from build123d import *

# Parameters (mm, degrees)
SKETCH1_W                = 10
SKETCH1_H                = 18
BOSS_EXTRUDE1_DEPTH      = 10
BOSS_EXTRUDE1_DEPTH_BACK = 10
SKETCH2_W                = 20
SKETCH2_H                = 2
BOSS_EXTRUDE2_DEPTH      = 20
SKETCH3_W                = 7
SKETCH3_H                = 4
SKETCH3_H_2              = 3
BOSS_EXTRUDE3_DEPTH      = 40
SKETCH7_R                = 1.5
CUT_EXTRUDE2_DEPTH       = 10


with BuildPart() as part:
    # Sketch1 → Boss-Extrude1 (new body, two sides)
    with BuildSketch(Plane.XY) as boss_extrude1_sk:
        with Locations((0, 6)):
            Rectangle(SKETCH1_W, SKETCH1_H)
    extrude(amount=BOSS_EXTRUDE1_DEPTH)
    extrude(boss_extrude1_sk.sketch, amount=-BOSS_EXTRUDE1_DEPTH_BACK)

    # Sketch2 → Boss-Extrude2 (add)
    with BuildSketch(Plane(origin=(0, 0, 0), x_dir=(0, 0, -1), z_dir=(1, 0, 0))):
        with Locations((0, -2)):
            Rectangle(SKETCH2_W, SKETCH2_H)
    extrude(amount=-BOSS_EXTRUDE2_DEPTH)

    # Sketch3 → Boss-Extrude3 (add)
    with BuildSketch(Plane(origin=(0, 0, 0), x_dir=(0, 0, -1), z_dir=(1, 0, 0))):
        with Locations((-6.5, 13)):
            Rectangle(SKETCH3_W, SKETCH3_H)
        with Locations((-6.5, -1.5)):
            Rectangle(SKETCH3_W, SKETCH3_H_2)
        with Locations((6.5, -1.5)):
            Rectangle(SKETCH3_W, SKETCH3_H_2)
        with Locations((6.5, 13)):
            Rectangle(SKETCH3_W, SKETCH3_H)
    extrude(amount=BOSS_EXTRUDE3_DEPTH)

    # Sketch7 → Cut-Extrude2 (cut)
    with BuildSketch(Plane(origin=(0, 0, 0), x_dir=(1, 0, 0), z_dir=(0, 1, 0))):
        with Locations((-12.5, 5)):
            Circle(SKETCH7_R)
        with Locations((-12.5, -5)):
            Circle(SKETCH7_R)
    extrude(amount=-CUT_EXTRUDE2_DEPTH, mode=Mode.SUBTRACT)


solid = part.part
Check sheet for the modelled part. Datum: model origin and axes. Units: mm. A direction names the side the tool comes from. Round coordinates to 2 decimals unless told otherwise and drop trailing zeros. Order: outer loops, then holes, each group sorted by start corner. A loop starts at its lowest first (then second) coordinate and runs counter-clockwise, first axis right, second up. Notation, with made-up numbers: M 39,-32 L 91,-32 A23 ccw 91,4 Z; hole C 21,-13.75 d3. An arc over 180 degrees is marked long. One line per item, written item: value. Start each with the question number.
1. Section check D-D on z = 7.5. Enter the section's corners in (x, y), and give its area (3 significant figures).
2. Section check A-A on x = 35. Enter the section's corners in (y, z), and give its area (3 significant figures).
3. Release check for a two-part mould opening along X. For faces 1 (the flat face through (10, 12, 10)), 2 (the cylindrical face through (-14, -2, -5)), 3 (the flat face through (40, -1, 7)) record: released by +X, released by -X, zero draft, split by the parting line, or undercut.
4. Section check B-B on z = -5. Enter the section's corners in (x, y), and give its area (3 significant figures).
5. Access from +Z, -Z, +X, -X, +Y, -Y to the whole of each face (thin tool, end or side, straight path). Record for faces 4 (the flat face through (22, 0, 7)), 5 (the flat face through (-5, 7, 0)), 6 (the flat face through (10, 12, -10)), 7 (the flat face through (22, -2, 3)).
6. Gauge pin test, flat ends, axial feed: P1, Ø2.5, axis at x = -12.5, z = -5, coming from the -Y side; P2, Ø2, axis at y = 12.5, z = -0.5, coming from the +X side; P3, Ø7.5, axis at x = -15, z = -2, coming from the +Y side. Record the tip position at first contact, or that the pin passes through.
7. Scan lines: line 1 along Z through (x, y) = (-12.5, -2.4); line 2 along X through (y, z) = (-2.5, 5); line 3 along Z through (x, y) = (26, 12.5). Record each from-to range of solid material in increasing order.
8. Section check C-C on x = -12.5. Enter the section's corners in (y, z).
Results found:
1. outline: M -20,-3 L 40,-3 L 40,0 L 5,0 L 5,11 L 40,11 L 40,15 L -5,15 L -5,-1 L -20,-1 Z
1. area: 455 mm^2
2. outline: M -3,-10 L 0,-10 L 0,-3 L -3,-3 Z; M -3,3 L 0,3 L 0,10 L -3,10 Z; M 11,-10 L 15,-10 L 15,-3 L 11,-3 Z; M 11,3 L 15,3 L 15,10 L 11,10 Z
2. area: 98.0 mm^2
3. face 1: zero draft
3. face 2: undercut
3. face 3: released by +X
4. outline: M -20,-3 L -14,-3 L -14,-1 L -20,-1 Z; M -11,-3 L 40,-3 L 40,0 L 5,0 L 5,11 L 40,11 L 40,15 L -5,15 L -5,-1 L -11,-1 Z
4. area: 449 mm^2
5. face 4: +Z, -Z, +X
5. face 5: +Z, -Z, -X, +Y
5. face 6: -Z, +X, -X, +Y, -Y
5. face 7: +X, +Y, -Y
6. P1: through
6. P2: x = 5
6. P3: y = -1
7. line 1: -10 to -6.5, -3.5 to 3.5, 6.5 to 10
7. line 2: -20 to -14, -11 to 40
7. line 3: -10 to -3, 3 to 10
8. outline: M -3,-10 L -1,-10 L -1,-6.5 L -3,-6.5 Z; M -3,-3.5 L -1,-3.5 L -1,3.5 L -3,3.5 Z; M -3,6.5 L -1,6.5 L -1,10 L -3,10 Z
